The listing builds one solid part. Answer for the finished solid, in the listing's coordinates (mm). Face numbers are marked on the shaded views. A direction names the side the tool comes from. Coordinates: 2 decimals unless noted, no trailing zeros. Loops run counter-clockwise (first coordinate to the right, second up) from the corner with the lowest first, then second, coordinate; pieces in that order, holes last. Notation, with made-up numbers: (-37, 48) -> (17, 48) arc R9 ccw to (17, 63) -> close; hole circle Ø5 at (75.25, 22.25). An arc over 180 degrees is marked (long way). Answer in a Markdown table with one row per item.
```python
from build123d import *

# Parameters (mm, degrees)
BOSS_EXTRUDE1_DEPTH = 25


with BuildPart() as part:
    # Sketch1 → Boss-Extrude1 (new body)
    with BuildSketch(Plane.XY):
        Polygon((-20, 0), (-10, 20), (0, 10), (0, 0), (-10, 10), align=None)
    extrude(amount=BOSS_EXTRUDE1_DEPTH)


solid = part.part
```
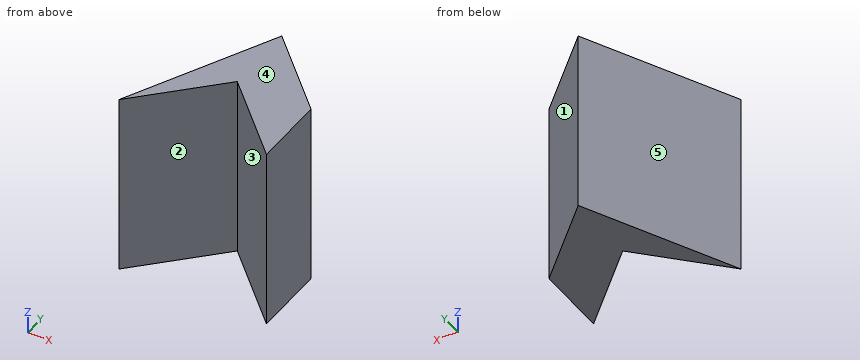
Item 1: A cutting plane is placed at D-D, the plane x = -18. Determine the outline of the cut face in (y, z).
Findings below:
| item | result |
|---|---|
| outline | (2, 0) -> (4, 0) -> (4, 25) -> (2, 25) -> close |
Item 2: Find the intervals of material crossed by probe 1 along X at (y, z) = (5.25, 8.5) (3 decimals); probe 2 along X at (y, z) = (6, 3); probe 3 along Y at (x, z) = (-9.5, 2.25), in increasing order.
Findings below:
| item | result |
|---|---|
| probe 1 | x = -17.375 to -14.75, -5.25 to 0 |
| probe 2 | x = -17 to -14, -6 to 0 |
| probe 3 | y = 9.5 to 19.5 |
Item 3: Flat-ended cylindrical pins translate along their axes: pin 1 Ø1 at (x, z) = (-10, 11) entering from -Y; pin 2 Ø1 at (y, z) = (2, 18) entering from -X; pin 3 Ø2 at (x, z) = (-10.5, 10) entering from -Y; pin 4 Ø8 at (y, z) = (8, 18) entering from +X. Find the tip coordinate at first contact, or state that the pin passes through.
Findings below:
| item | result |
|---|---|
| pin 1 | stops at y = 9.5 |
| pin 2 | stops at x = -19.25 |
| pin 3 | stops at y = 8.5 |
| pin 4 | stops at x = 0 |
Item 4: A cutting plane is placed at C-C, the plane z = 11.75. Determine the outline of the cut face in (x, y).
Findings below:
| item | result |
|---|---|
| outline | (-20, 0) -> (-10, 10) -> (0, 0) -> (0, 10) -> (-10, 20) -> close |
Item 5: Determine the mould class of the marked faces 3, 4 and 5 for opening direction X: +X half, -X half, draft (parallel to the pull), parting line (faces both ways), or undercut.
Findings below:
| item | result |
|---|---|
| face 3 | undercut |
| face 4 | draft |
| face 5 | -X half |
Item 6: A tool of negligible diameter and unlimited length cuts with its end or side. For the marked faces 1 and 2, from which of +Z, -Z, +X, -X, +Y, -Y can it reach the whole face along a straight path? Write none if from no direction.
Findings below:
| item | result |
|---|---|
| face 1 | +Z, -Z, +X, +Y |
| face 2 | +Z, -Z, -Y |
Item 7: A cutting plane is placed at B-B, the plane y = 9. Determine the outline of the cut face in (x, z).
Findings below:
| item | result |
|---|---|
| outline | (-15.5, 0) -> (-11, 0) -> (-11, 25) -> (-15.5, 25) -> close; (-9, 0) -> (0, 0) -> (0, 25) -> (-9, 25) -> close |
Item 8: A cutting plane is placed at A-A, the plane y = 3.5. Determine the outline of the cut face in (x, z).
Findings below:
| item | result |
|---|---|
| outline | (-18.25, 0) -> (-16.5, 0) -> (-16.5, 25) -> (-18.25, 25) -> close; (-3.5, 0) -> (0, 0) -> (0, 25) -> (-3.5, 25) -> close |
